```python
from build123d import *

# Parameters (mm, degrees)
SKETCH1_W                 = 180
SKETCH1_H                 = 175
PLATE_DEPTH               = 6
FILLET_CORNERS_R          = 5
SKETCH2_R                 = 2.25
MOTOR_BRACKET_HOLES_DEPTH = 126.667219274
SKETCH3_R                 = 1.2
CASTER_HOLES_DEPTH        = 126.667219274
SKETCH4_R                 = 2.25
ULTRASOUND_HOLES_DEPTH    = 126.667219274
SKETCH6_R                 = 2.25
BATTERY_CAGE_HOLES_DEPTH  = 126.667219274
SKETCH5_R                 = 2.25
FRONT_HOLES_DEPTH         = 126.667219274
TEAM_NAME_DEPTH           = 0.25
SKETCH8_R                 = 1.6
BEACON_HOLES_DEPTH        = 126.667219415


with BuildPart() as part:
    # Sketch1 → plate (new body)
    with BuildSketch(Plane(origin=(0, 0, 0), x_dir=(1, 0, 0), z_dir=(0, 1, 0))):
        Rectangle(SKETCH1_W, SKETCH1_H)
    extrude(amount=PLATE_DEPTH)

    # Fillet corners
    fillet_corners_edges = [part.edges().sort_by_distance(p)[0] for p in [
        (-90, 3, -87.5),
        (90, 3, -87.5),
        (90, 3, 87.5),
        (-90, 3, 87.5),
    ]]
    fillet(fillet_corners_edges, radius=FILLET_CORNERS_R)

    # Sketch2 → motor bracket holes (cut, through all)
    with BuildSketch(Plane(origin=(0, 6, 0), x_dir=(1, 0, 0), z_dir=(0, 1, 0))):
        with Locations(Location((-77.5, 72.5, 0), (0, 0, 270))):
            Circle(SKETCH2_R)
        with Locations(Location((-42.5, 72.5, 0), (0, 0, 270))):
            Circle(SKETCH2_R)
        with Locations(Location((-42.5, 47.5, 0), (0, 0, 270))):
            Circle(SKETCH2_R)
        with Locations(Location((-77.5, 47.5, 0), (0, 0, 270))):
            Circle(SKETCH2_R)
    motor_bracket_holes = extrude(amount=-MOTOR_BRACKET_HOLES_DEPTH, mode=Mode.SUBTRACT)

    # Sketch3 → caster holes (cut, through all)
    with BuildSketch(Plane(origin=(0, 6, 0), x_dir=(1, 0, 0), z_dir=(0, 1, 0))):
        with Locations(Location((-7.75, -75.5, 0), (0, 0, 270))):
            Circle(SKETCH3_R)
        with Locations(Location((7.75, -75.5, 0), (0, 0, 270))):
            Circle(SKETCH3_R)
    extrude(amount=-CASTER_HOLES_DEPTH, mode=Mode.SUBTRACT)

    # Sketch4 → ultrasound holes (cut, through all)
    with BuildSketch(Plane(origin=(0, 6, 0), x_dir=(1, 0, 0), z_dir=(0, 1, 0))):
        with Locations(Location((-80, -52.5, 0), (0, 0, 270))):
            Circle(SKETCH4_R)
        with Locations(Location((-80, -27.5, 0), (0, 0, 270))):
            Circle(SKETCH4_R)
    ultrasound_holes = extrude(amount=-ULTRASOUND_HOLES_DEPTH, mode=Mode.SUBTRACT)

    # Sketch6 → battery cage holes (cut, through all)
    with BuildSketch(Plane(origin=(0, 6, 0), x_dir=(1, 0, 0), z_dir=(0, 1, 0))):
        with Locations(Location((-25, -80, 0), (0, 0, 270))):
            Circle(SKETCH6_R)
    battery_cage_holes = extrude(amount=-BATTERY_CAGE_HOLES_DEPTH, mode=Mode.SUBTRACT)

    # Sketch5 → front holes (cut, through all)
    with BuildSketch(Plane(origin=(0, 6, 0), x_dir=(1, 0, 0), z_dir=(0, 1, 0))):
        with Locations(Location((-15, 77.5, 0), (0, 0, 270))):
            Circle(SKETCH5_R)
        with Locations(Location((15, 77.5, 0), (0, 0, 270))):
            Circle(SKETCH5_R)
    extrude(amount=-FRONT_HOLES_DEPTH, mode=Mode.SUBTRACT)

    # Mirror holes: motor bracket holes, ultrasound holes, battery cage holes across plane
    add(motor_bracket_holes.mirror(Plane(origin=(0, 0, 0), x_dir=(0, 0, 1), z_dir=(1, 0, 0))), mode=Mode.SUBTRACT)
    add(ultrasound_holes.mirror(Plane(origin=(0, 0, 0), x_dir=(0, 0, 1), z_dir=(1, 0, 0))), mode=Mode.SUBTRACT)
    add(battery_cage_holes.mirror(Plane(origin=(0, 0, 0), x_dir=(0, 0, 1), z_dir=(1, 0, 0))), mode=Mode.SUBTRACT)

    # Sketch7 → team name (cut)
    with BuildSketch(Plane(origin=(0, 6, 0), x_dir=(1, 0, 0), z_dir=(0, 1, 0))):
        Polygon((41.490517689, -79.14413255), (42.552216407, -29.14413255), (43.123129869, -29.14413255), (46.939235638, -71.061199858), (50.825453587, -29.14413255), (51.306222818, -29.14413255), (52.387953587, -79.14413255), (51.756943972, -79.14413255), (50.785389484, -41.694212678), (47.269764484, -79.14413255), (46.618722818, -79.14413255), (43.093081792, -41.64413255), (42.121527305, -79.14413255), align=None)
        Polygon((53.776174741, -29.14413255), (55.208466407, -29.14413255), (55.208466407, -79.14413255), (54.567440766, -79.14413255), (54.567440766, -34.272337678), (53.285389484, -34.272337678), align=None)
        Polygon((59.160790125, -29.14413255), (60.593081792, -29.14413255), (60.593081792, -79.14413255), (59.952056151, -79.14413255), (59.952056151, -34.272337678), (58.670004869, -34.272337678), align=None)
        with BuildLine():
            Line((63.413594613, -44.528747935), (62.772568972, -44.528747935))
            add(Edge.make_bspline(
                [(62.772568972, -44.528747935), (62.781493316, -43.93445176), (62.798943386, -42.772404539), (62.842798919, -41.072258174), (62.935478667, -39.452750644), (63.05750017, -37.917150742), (63.19141105, -36.456345848), (63.373095419, -35.080629373), (63.581991977, -33.784289246), (63.820632002, -32.581935586), (64.074552978, -31.491828406), (64.344756451, -30.540110197), (64.61215525, -29.731836807), (64.884672979, -29.067522721), (65.17629041, -28.549168463), (65.459482684, -28.166880995), (65.766362376, -27.911333409), (65.994533796, -27.877435937), (66.097889484, -27.862081268)],
                knots=[0, 0, 0, 0, 1.632956762, 3.192975066, 4.67207115, 6.088935359, 7.425149098, 8.701691951, 9.900535109, 11.032042853, 12.068832046, 12.974740653, 13.7492155, 14.406834829, 14.944978755, 15.376189076, 15.717429958, 16, 16, 16, 16], degree=3))
            add(Edge.make_bspline(
                [(66.097889484, -27.862081268), (66.214593659, -27.876513312), (66.459978019, -27.906858394), (66.789228182, -28.148258945), (67.095157034, -28.504713995), (67.376289014, -29.00124848), (67.646270357, -29.629255057), (67.889389184, -30.396480918), (68.13076794, -31.297967968), (68.422485253, -32.715843502), (68.730325215, -34.671525798), (68.998284034, -37.188458627), (69.158674349, -39.905916797), (69.174590453, -41.784130898), (69.182825382, -42.755911396)],
                knots=[0, 0, 0, 0, 0.265111354, 0.557428048, 0.903723158, 1.338574996, 1.855033468, 2.4660581, 3.177426512, 3.989273206, 5.775956304, 7.703955125, 9.777243485, 12, 12, 12, 12], degree=3))
            add(Edge.make_bspline(
                [(69.182825382, -42.755911396), (69.174478109, -43.45049961), (69.15801384, -44.820514374), (69.047340862, -46.842189249), (68.862186477, -48.797931916), (68.622075004, -50.396898082), (68.411616198, -51.695290325), (68.214396392, -52.741857038), (68.009797757, -53.872058653), (67.763428304, -55.085556549), (67.507271104, -56.381810617), (67.222599468, -57.759829632), (66.926861643, -59.220525286), (66.710071993, -60.220774042), (66.598690766, -60.734677422)],
                knots=[0, 0, 0, 0, 1.373593798, 2.709294146, 4.002897475, 5.256921411, 5.906027412, 6.604062607, 7.36293037, 8.177408102, 9.052743955, 9.975998375, 10.960117401, 12, 12, 12, 12], degree=3))
            Line((66.598690766, -60.734677422), (63.834267689, -74.015927422))
            Line((63.834267689, -74.015927422), (69.182825382, -74.015927422))
            Line((69.182825382, -74.015927422), (69.182825382, -79.14413255))
            Line((69.182825382, -79.14413255), (62.13154333, -79.14413255))
            Line((62.13154333, -79.14413255), (66.438434356, -58.451023576))
            add(Edge.make_bspline(
                [(66.438434356, -58.451023576), (66.541275625, -57.956765987), (66.740022638, -57.001583104), (67.038126467, -55.62227416), (67.281204083, -54.337396726), (67.517596013, -53.153963402), (67.714834282, -52.068252304), (67.888303774, -51.080497667), (68.028581018, -50.192251945), (68.246517983, -48.62036821), (68.489685546, -46.278314551), (68.524176548, -44.192336007), (68.541799741, -43.126504345)],
                knots=[0, 0, 0, 0, 0.977048528, 1.888205767, 2.730899807, 3.507700373, 4.223757048, 4.86643668, 5.448577838, 5.963957604, 7.937782349, 10, 10, 10, 10], degree=3))
            add(Edge.make_bspline(
                [(68.541799741, -43.126504345), (68.536927467, -42.458412904), (68.527536358, -41.170693779), (68.377133023, -39.312911942), (68.172341189, -37.593632449), (67.892830311, -36.269968348), (67.657192593, -35.307097273), (67.453256742, -34.701856907), (67.260548337, -34.179683247), (67.036846336, -33.761564083), (66.823881555, -33.42188765), (66.588014894, -33.178683952), (66.333600869, -33.026029048), (66.152915281, -33.001728194), (66.067841407, -32.990286396)],
                knots=[0, 0, 0, 0, 2.216081534, 4.27140717, 6.18139161, 7.956427784, 8.757128989, 9.468293711, 10.075172411, 10.600423608, 11.039796501, 11.400135884, 11.717560408, 12, 12, 12, 12], degree=3))
            add(Edge.make_bspline(
                [(66.067841407, -32.990286396), (65.976155684, -33.00133342), (65.785870557, -33.024260481), (65.514038504, -33.177258474), (65.276430893, -33.434342115), (65.034037095, -33.763688283), (64.817075996, -34.1957923), (64.608254954, -34.718950361), (64.4125659, -35.339425303), (64.222521115, -36.047247528), (64.054411991, -36.839902752), (63.905399587, -37.712091101), (63.776129767, -38.660944953), (63.670442917, -39.686954193), (63.563011117, -40.787882759), (63.503471574, -41.967808104), (63.434232438, -43.222631631), (63.420612628, -44.084595296), (63.413594613, -44.528747935)],
                knots=[0, 0, 0, 0, 0.357691352, 0.74235488, 1.184483885, 1.716016461, 2.333635849, 3.0641575, 3.912772014, 4.870186639, 5.9228254, 7.072838979, 8.321875155, 9.658267009, 11.097074475, 12.63688611, 14.267054667, 16, 16, 16, 16], degree=3))
        make_face()
    extrude(amount=-TEAM_NAME_DEPTH, mode=Mode.SUBTRACT)

    # Sketch8 → beacon holes (cut, through all)
    with BuildSketch(Plane(origin=(0, 6, 0), x_dir=(1, 0, 0), z_dir=(0, 1, 0))):
        with Locations(Location((0, 45, 0), (0, 0, 270))):
            Circle(SKETCH8_R)
        with Locations(Location((0, 60, 0), (0, 0, 270))):
            Circle(SKETCH8_R)
    extrude(amount=-BEACON_HOLES_DEPTH, mode=Mode.SUBTRACT)


solid = part.part
```
For this review, take the finished solid that the model builds, in its own axes (mm). A direction names the side the tool comes from. Coordinates: 2 decimals unless noted, no trailing zeros. Loops run counter-clockwise (first coordinate to the right, second up) from the corner with the lowest first, then second, coordinate; pieces in that order, holes last.
1. For line 1 (X direction, y = 4.75, z = -72.5); line 2 (X direction, y = 1.9, z = 75.5); line 3 (Z direction, x = 80, y = 4.85), list the stretches that pass through material, from the lowest coordinate up.
2. Add section A-A, the plane x = 15. Give the boundary of the cut face in (y, z).
3. Mouldability with a two-part tool opening along X and no side actions: class faces 1 (the cylindrical face through (-15.86, 3.04, -75.42)), 2 (the cylindrical face through (-82.196, 3.042, 27.012)), 3 (the flat face through (-1, 3, 87.5)), 4 (the cylindrical face through (-88.57, 3.04, 86)) as +X half, -X half, draft (parallel to the pull), parting line (faces both ways), or undercut.
4. Insertion check: P1, Ø4, axis at x = -80, z = 27.5, coming from the +Y side. The pin has a flat end and moves straight along its axis. Give the tip position at first contact, or say it passes through.
5. For faces 5 (the flat face through (45, 5.75, 54)), 6 (the cylindrical face through (-79.496, 3.042, -71.462)), list the 3-axis set-ups (+Z, -Z, +X, -X, +Y, -Y) from which the entire face can be reached by the end or side of a thin tool; tool diameter is ignored.
Result:
1. line 1: x = -90 to -79.75, -75.25 to -44.75, -40.25 to 40.25, 44.75 to 75.25, 79.75 to 90
1. line 2: x = -90 to -8.95, -6.55 to 6.55, 8.95 to 90
1. line 3: z = -87.5 to 25.25, 29.75 to 50.25, 54.75 to 87.5
2. outline: (0, -87.5) - (6, -87.5) - (6, -79.75) - (0, -79.75) - close; (0, -75.25) - (6, -75.25) - (6, 87.5) - (0, 87.5) - close
3. face 1: undercut
3. face 2: undercut
3. face 3: draft
3. face 4: -X half
4. P1: passes through
5. face 5: +Y
5. face 6: +Y, -Y
